```python
from build123d import *

# Parameters (mm, degrees)
BOSS_EXTRUDE1_DEPTH = 5
SKETCH3_W           = 5
SKETCH3_H           = 15
BOSS_EXTRUDE2_DEPTH = 5
CUT_EXTRUDE2_DEPTH  = 5
SKETCH5_R           = 1.5
CUT_EXTRUDE3_DEPTH  = 5


with BuildPart() as part:
    # Sketch1 → Boss-Extrude1 (new body)
    with BuildSketch(Plane.XY):
        Polygon((0, 31.783783784), (10, 31.783783784), (40, 31.783783784), (40, 21.783783784), (40, -48.216216216), (-40, -48.216216216), (-40, 31.783783784), align=None)
    extrude(amount=BOSS_EXTRUDE1_DEPTH)

    # Sketch3 → Boss-Extrude2 (add)
    with BuildSketch(Plane.ZY.offset(40)):
        with Locations((2.5, 9.283783784)):
            Rectangle(SKETCH3_W, SKETCH3_H)
        with Locations((2.5, -25.716216216)):
            Rectangle(SKETCH3_W, SKETCH3_H)
    extrude(amount=BOSS_EXTRUDE2_DEPTH)

    # Sketch4 → Cut-Extrude2 (cut)
    with BuildSketch(Plane.XY.offset(5)):
        Polygon((-40, 31.783783784), (-25, 31.783783784), (-40, 24.283783784), align=None)
        Polygon((-40, -48.216216216), (-40, -40.716216216), (-25, -48.216216216), align=None)
    extrude(amount=-CUT_EXTRUDE2_DEPTH, mode=Mode.SUBTRACT)

    # Sketch5 → Cut-Extrude3 (cut)
    with BuildSketch(Plane.XY.offset(5)):
        with Locations((30, 1.783783784)):
            Circle(SKETCH5_R)
    extrude(amount=-CUT_EXTRUDE3_DEPTH, mode=Mode.SUBTRACT)


solid = part.part
```
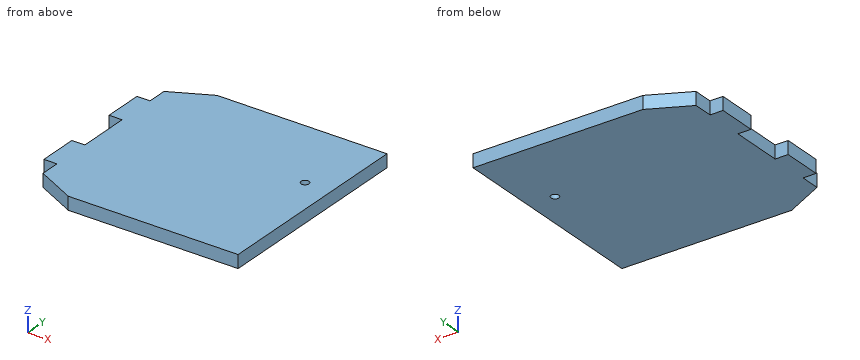
Check sheet for the modelled part. Datum: model origin and axes. Units: mm. Coordinates: 2 decimals unless noted, no trailing zeros. Write each loop counter-clockwise with the first axis right and the second up, starting at its lowest first coordinate (ties: lowest second). Pieces come first, ordered by that corner, then holes. Notation, with made-up numbers: (54, 4) -> (73, 4) arc R27 cw to (73, 22) -> close; hole circle Ø2 at (77.25, 17). An arc over 180 degrees is marked (long way). Use a Markdown table: item, result.
1. Sectioned sample at D-D (x = -33). Enter the section's corners in (y, z), plus the area to 3 significant figures.
Reported:
| item | result |
|---|---|
| outline | (-44.22, 0) -> (27.78, 0) -> (27.78, 5) -> (-44.22, 5) -> close |
| area | 360 mm2 |
2. Sectioned sample at A-A (x = 30). Enter the section's corners in (y, z).
Reported:
| item | result |
|---|---|
| outline | (-48.22, 0) -> (0.28, 0) -> (0.28, 5) -> (-48.22, 5) -> close; (3.28, 0) -> (31.78, 0) -> (31.78, 5) -> (3.28, 5) -> close |
3. Sectioned sample at B-B (z = 1.35). Enter the section's corners in (x, y), plus the area to 3 significant figures.
Reported:
| item | result |
|---|---|
| outline | (-45, -33.22) -> (-40, -33.22) -> (-40, -40.72) -> (-25, -48.22) -> (40, -48.22) -> (40, 31.78) -> (-25, 31.78) -> (-40, 24.28) -> (-40, 16.78) -> (-45, 16.78) -> (-45, 1.78) -> (-40, 1.78) -> (-40, -18.22) -> (-45, -18.22) -> close; hole circle Ø3 at (30, 1.78) |
| area | 6,430 mm2 |
4. Sectioned sample at C-C (y = -7). Enter the section's corners in (x, z).
Reported:
| item | result |
|---|---|
| outline | (-40, 0) -> (40, 0) -> (40, 5) -> (-40, 5) -> close |
5. Scan lines: line 1 along Y through (x, z) = (-40.5, 4.7); line 2 along Y through (x, z) = (30, 3); line 3 along X through (y, z) = (2, 3.5). Record each from-to range of solid material in increasing order.
Reported:
| item | result |
|---|---|
| line 1 | y = -33.22 to -18.22, 1.78 to 16.78 |
| line 2 | y = -48.22 to 0.28, 3.28 to 31.78 |
| line 3 | x = -45 to 28.52, 31.48 to 40 |
6. Go/stop test with flat-tipped pins: pin 1 Ø1.5 at (y, z) = (-36.5, 1.5) entering from -X; pin 2 Ø1.5 at (x, z) = (-43.5, 2.5) entering from -Y; pin 3 Ø1.5 at (x, z) = (-41.5, 3.5) entering from +Y. Record where each tip stops, or that it passes through.
Reported:
| item | result |
|---|---|
| pin 1 | stops at x = -40 |
| pin 2 | stops at y = -33.22 |
| pin 3 | stops at y = 16.78 |
